from build123d import *

# Parameters (mm, degrees)
SKETCH_1_W          = 75
SKETCH_1_H          = 20
EXTRUDE_1_DEPTH     = 5
SKETCH_2_R          = 1.5
CUT_EXTRUDE_1_DEPTH = 40.131189606
CUT_EXTRUDE_2_DEPTH = 40.131189606


with BuildPart() as part:
    # 草图1 → 凸台-拉伸1 (new body)
    with BuildSketch(Plane(origin=(0, 0, 0), x_dir=(1, 0, 0), z_dir=(0, 1, 0))):
        Rectangle(SKETCH_1_W, SKETCH_1_H)
    extrude(amount=EXTRUDE_1_DEPTH)

    # 草图2 → 切除-拉伸1 (cut, through all)
    with BuildSketch(Plane(origin=(0, 5, 0), x_dir=(1, 0, 0), z_dir=(0, 1, 0))):
        with Locations(Location((22.5, 5, 0), (0, 0, 270))):
            Circle(SKETCH_2_R)
        with Locations(Location((32.5, 5, 0), (0, 0, 270))):
            Circle(SKETCH_2_R)
        with Locations(Location((22.5, -5, 0), (0, 0, 270))):
            Circle(SKETCH_2_R)
        with Locations(Location((32.5, -5, 0), (0, 0, 270))):
            Circle(SKETCH_2_R)
    cut_extrude_1 = extrude(amount=-CUT_EXTRUDE_1_DEPTH, mode=Mode.SUBTRACT)

    # 草图3 → 切除-拉伸2 (cut, through all)
    with BuildSketch(Plane(origin=(0, 5, 0), x_dir=(1, 0, 0), z_dir=(0, 1, 0))):
        with BuildLine():
            Line((6.81829997, -5.602297427), (-6.81829997, -5.602297427))
            ThreePointArc((-6.81829997, -5.602297427), (-12.420597397, 0), (-6.81829997, 5.602297427))
            Line((-6.81829997, 5.602297427), (6.81829997, 5.602297427))
            ThreePointArc((6.81829997, 5.602297427), (12.420597397, 0), (6.81829997, -5.602297427))
        make_face()
    extrude(amount=-CUT_EXTRUDE_2_DEPTH, mode=Mode.SUBTRACT)

    # 镜向1: 切除-拉伸1 across plane
    add(cut_extrude_1.mirror(Plane(origin=(0, 0, 0), x_dir=(0, 0, 1), z_dir=(1, 0, 0))), mode=Mode.SUBTRACT)


solid = part.part
Design review of the part built by this model. Coordinates are the model's own, in mm. A direction names the side the tool comes from. Round coordinates to 2 decimals unless told otherwise and drop trailing zeros. Loops run counter-clockwise (first coordinate to the right, second up) from the corner with the lowest first, then second, coordinate; pieces in that order, holes last. Notation, with made-up numbers: M 46,-22.75 L 68,-22.75 A10 ccw 68,-5.75 Z; hole C 33.25,-34 d4. An arc over 180 degrees is marked long. Answer as a JSON object with one key per item and string values.
Item 1: Wall thickness on L1, parallel to Z at x = -32.5, y = 3.45; L2, parallel to Z at x = -4.5, y = 2.3; L3, parallel to Z at x = 32, y = 3.05: over which ranges is each line inside the solid? List them lowest first. Write a range as from..to.
Answer sheet:
{"L1": "z = -10..-6.5, -3.5..3.5, 6.5..10", "L2": "z = -10..-5.6, 5.6..10", "L3": "z = -10..-6.41, -3.59..3.59, 6.41..10"}
Item 2: We need section A-A on x = -0.5. Give the boundary of the cut face in (y, z), and give its area (3 significant figures).
Answer sheet:
{"outline": "M 0,-10 L 5,-10 L 5,-5.6 L 0,-5.6 Z; M 0,5.6 L 5,5.6 L 5,10 L 0,10 Z", "area": "44.0 mm^2"}
Item 3: We need section B-B on z = 0. Give the boundary of the cut face in (x, y), and give its area (3 significant figures).
Answer sheet:
{"outline": "M -37.5,0 L -12.42,0 L -12.42,5 L -37.5,5 Z; M 12.42,0 L 37.5,0 L 37.5,5 L 12.42,5 Z", "area": "251 mm^2"}
Item 4: We need section C-C on y = 4.15. State how many separate pieces and enclosed holes the cut face has, and give its area (3 significant figures).
Answer sheet:
{"separate pieces": "1", "enclosed holes": "9", "area": "1,190 mm^2"}
Item 5: We need section D-D on x = 22.5. Give the boundary of the cut face in (y, z), and give its area (3 significant figures).
Answer sheet:
{"outline": "M 0,-10 L 5,-10 L 5,-6.5 L 0,-6.5 Z; M 0,-3.5 L 5,-3.5 L 5,3.5 L 0,3.5 Z; M 0,6.5 L 5,6.5 L 5,10 L 0,10 Z", "area": "70.0 mm^2"}
Item 6: The part is to be moulded in two halves that separate along Z. For faces 1 (the flat face through (-1, 0, 7)), 2 (the flat face through (-1, 2, 10)), 3 (the cylindrical face through (23.765, 2.535, 5.806)), say which applies: pulls with the +Z half, pulls with the -Z half, needs draft (parallel to the pull), parting line crosses it, or undercut.
Answer sheet:
{"face 1": "needs draft", "face 2": "pulls with the +Z half", "face 3": "undercut"}
Item 7: Machinability: for faces 4 (the flat face through (0, 3, 5.602)), 5 (the flat face through (37.5, 2, 0)), which of the approach directions +Z, -Z, +X, -X, +Y, -Y give a long, thin tool a straight path to every point of the face, cutting with its end or side? Answer none if there is none.
Answer sheet:
{"face 4": "+Y, -Y", "face 5": "+Z, -Z, +X, +Y, -Y"}
